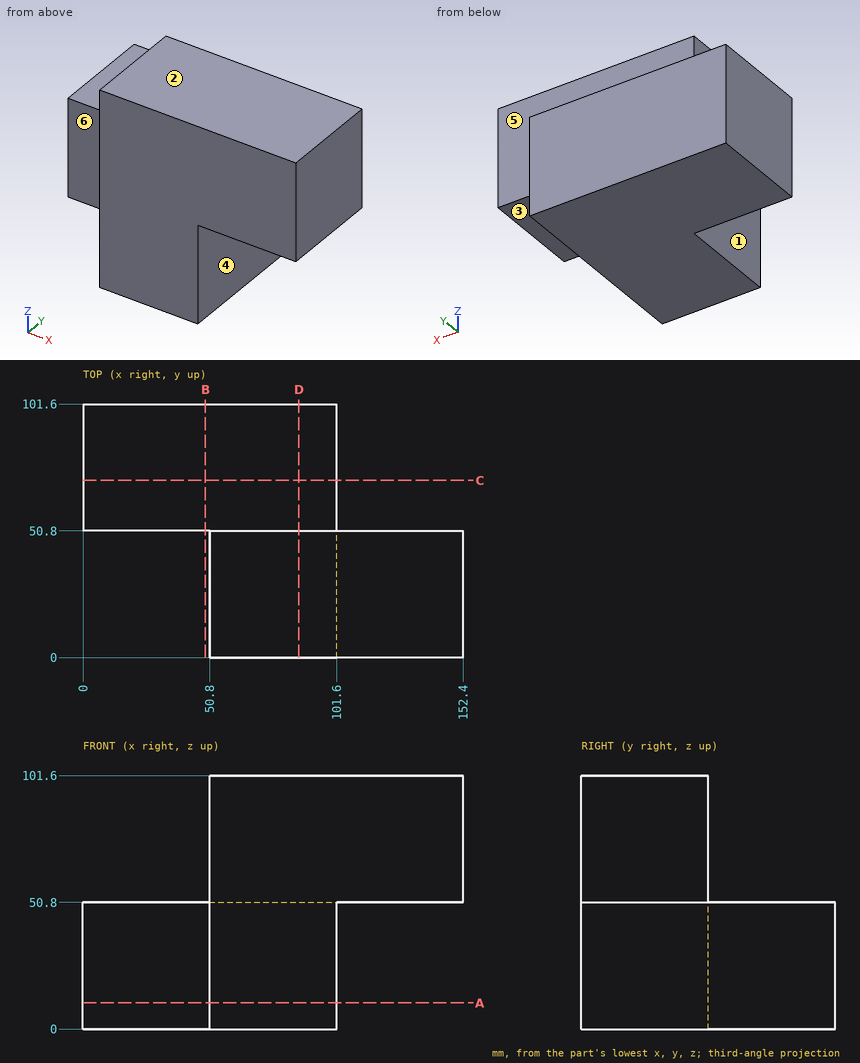
The figure shows three views and two pictorial views of one solid part (mm, origin at its lowest corner). Answer the questions. A direction names the side the tool comes from. Round coordinates to 2 decimals unless told otherwise and drop trailing zeros. Write each loop counter-clockwise with the first axis right and the second up, starting at its lowest first coordinate (ties: lowest second). Pieces come first, ordered by that corner, then holes. Notation, with made-up numbers: M -4,-21 L 35,-21 A34 cw 35,17 Z; hole C 34,15 d2. An arc over 180 degrees is marked long. Use a Markdown table: item, result.
1) The part is cut by section A-A on z = 10.5. Give the vertices of the cut face in (x, y).
Taken from the geometry:
| item | result |
|---|---|
| outline | M 0,50.8 L 50.8,50.8 L 50.8,0 L 101.6,0 L 101.6,101.6 L 0,101.6 Z |
2) The part is cut by section D-D on x = 86.5. Give the vertices of the cut face in (y, z), plus the area to 3 significant figures.
Taken from the geometry:
| item | result |
|---|---|
| outline | M 0,0 L 101.6,0 L 101.6,50.8 L 50.8,50.8 L 50.8,101.6 L 0,101.6 Z |
| area | 7,740 mm2 |
3) The part is cut by section C-C on y = 71. Give the vertices of the cut face in (x, z).
Taken from the geometry:
| item | result |
|---|---|
| outline | M 0,0 L 101.6,0 L 101.6,50.8 L 0,50.8 Z |
4) Consider line 1 (X direction, y = 14.5, z = 71.5); line 2 (Z direction, x = 6.5, y = 89). Determine where each line is inside the solid, lowest interval first. Write a range as [from, to].
Taken from the geometry:
| item | result |
|---|---|
| line 1 | x = [50.8, 152.4] |
| line 2 | z = [0, 50.8] |
5) Which of the six approach directions +Z, -Z, +X, -X, +Y, -Y give full straight-line access (tool end or side, diameter ignored) to the marked faces 4, 5 and 6?
Taken from the geometry:
| item | result |
|---|---|
| face 4 | -Z, +X, +Y, -Y |
| face 5 | +Z, +X, -X, +Y |
| face 6 | +Z, -Z, -X, -Y |
6) Determine the mould class of the marked faces 1, 2 and 3 for opening direction Z: pulls with the +Z half, pulls with the -Z half, needs draft (parallel to the pull), parting line crosses it, or undercut.
Taken from the geometry:
| item | result |
|---|---|
| face 1 | needs draft |
| face 2 | pulls with the +Z half |
| face 3 | pulls with the -Z half |
7) The part is cut by section B-B on x = 49. Give the vertices of the cut face in (y, z).
Taken from the geometry:
| item | result |
|---|---|
| outline | M 50.8,0 L 101.6,0 L 101.6,50.8 L 50.8,50.8 Z |
8) Flat-ended cylindrical pins translate along their axes: pin 1 (6 mm diameter, centred on x = 66, z = 57, fed in from +Y); pin 2 (15 mm diameter, centred on y = 35, z = 36, fed in from -X); pin 3 (8 mm diameter, centred on y = 50, z = 21.5, fed in from -X). Find the tip coordinate at first contact, or state that the pin passes through.
Taken from the geometry:
| item | result |
|---|---|
| pin 1 | stops at y = 50.8 |
| pin 2 | stops at x = 50.8 |
| pin 3 | stops at x = 0 |
